Read the model definition and answer for the solid it produces. Units are mm, in the model's axes. Face numbers are marked on the shaded views. A direction names the side the tool comes from. Give positions to 0.01 mm unless a question says otherwise; leave off trailing zeros. Order: outer loops, then holes, each group sorted by start corner. A loop starts at its lowest first (then second) coordinate and runs counter-clockwise, first axis right, second up. Notation, with made-up numbers: (58, 18) - (99, 18) arc R9 cw to (99, 29) - close; hole circle Ø10 at (12.25, 76). An arc over 180 degrees is marked (long way). One line per item, written item: value. Start each with the question number.
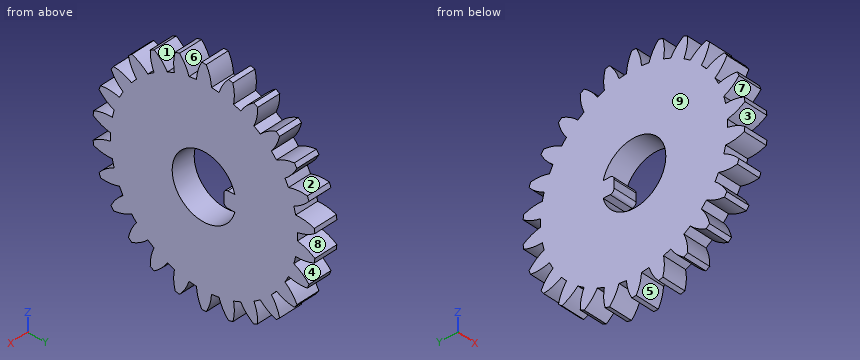
```python
from build123d import *

# Parameters (mm, degrees)
BASPROSKE_W                 = 3
BASPROSKE_H                 = 14
TOOTHCUT_DEPTH              = 21.024984395
TEETHCUTS_COUNT             = 26
TEETHCUTS_ANGLE             = 346.153846154
BORSKE_R                    = 4
BORE_DEPTH                  = 50.0000508
DODANIE_WYCI_GNI_CIE1_DEPTH = 3


with BuildPart() as part:
    # BasProSke → Base-Revolve (revolve)
    with BuildSketch(Plane(origin=(0, 0, 0), x_dir=(1, 0, 0), z_dir=(0, 1, 0)), mode=Mode.PRIVATE) as base_revolve_sk:
        with Locations((1.5, 7)):
            Rectangle(BASPROSKE_W, BASPROSKE_H)
    revolve(base_revolve_sk.sketch.rotate(Axis((-10, 0, 0), (1, 0, 0)), 180), axis=Axis((-10, 0, 0), (1, 0, 0)))

    # TooCutSke → ToothCut (cut, through all)
    with BuildSketch(Plane(origin=(0, 0, 0), x_dir=(0, 0, -1), z_dir=(1, 0, 0))):
        with BuildLine():
            ThreePointArc((0.476965065, 11.739314517), (0, 11.749), (-0.476965065, 11.739314517))
            ThreePointArc((-0.476965065, 11.739314517), (-0.82065865, 12.901686978), (-1.424117301, 13.952911348))
            ThreePointArc((-1.424117301, 13.952911348), (0, 14.0254), (1.424117301, 13.952911348))
            ThreePointArc((1.424117301, 13.952911348), (0.82065865, 12.901686978), (0.476965065, 11.739314517))
        make_face()
    toothcut = extrude(amount=TOOTHCUT_DEPTH, mode=Mode.SUBTRACT)

    # TeethCuts: ToothCut ×26 about axis
    teethcuts_axis = Axis((-10, 0, 0), (1, 0, 0))
    for i in range(1, TEETHCUTS_COUNT):
        add(toothcut.rotate(teethcuts_axis, i * TEETHCUTS_ANGLE / (TEETHCUTS_COUNT - 1)), mode=Mode.SUBTRACT)

    # BorSke → Bore (cut, symmetric)
    with BuildSketch(Plane(origin=(0, 0, 0), x_dir=(0, 0, -1), z_dir=(1, 0, 0))):
        with Locations(Location((0, 0, 0), (0, 0, 180))):
            Circle(BORSKE_R)
    extrude(amount=BORE_DEPTH, both=True, mode=Mode.SUBTRACT)

    # Szkic1 → Dodanie-wyciągnięcie1 (add)
    with BuildSketch(Plane(origin=(3, 0, 0), x_dir=(0, 0, -1), z_dir=(1, 0, 0))):
        with BuildLine():
            Line((0, 4), (-1, 4))
            Line((-1, 4), (-1, 3))
            ThreePointArc((-1, 3), (-0.853553391, 2.646446609), (-0.5, 2.5))
            Line((-0.5, 2.5), (0.5, 2.5))
            ThreePointArc((0.5, 2.5), (0.853553391, 2.646446609), (1, 3))
            Line((1, 3), (1, 4))
            Line((1, 4), (0, 4))
        make_face()
    extrude(amount=-DODANIE_WYCI_GNI_CIE1_DEPTH)


solid = part.part
```
1) Section A-A on z = 0 is taken. Write down the section's boundary in (x, y), plus the area to 3 significant figures.
2) Each of these flat-tipped pins is pushed along its axis until it touches: pin 1 (5 mm diameter, centred on y = 7, z = -5, fed in from -X); pin 2 (0.7 mm diameter, centred on x = 2, y = 3.5, fed in from -Z); pin 3 (0.8 mm diameter, centred on x = 1.5, z = 0, fed in from -Y); pin 4 (1 mm diameter, centred on x = 2, y = 3.5, fed in from +Z). Where does it stop, or does it pass through?
3) Section B-B on z = 6.5 is taken. Write down the section's boundary in (x, y), plus the area to 3 significant figures.
4) Section C-C on z = -7 is taken. Write down the section's boundary in (x, y), plus the area to 3 significant figures.
5) For the marked faces 1, 2, 3, 4 and 5, determine the directions among +Z, -Z, +X, -X, +Y, -Y from which every point of the face is accessible in a straight line to the end or side of a thin tool.
6) The mould has two halves that part along Y. Classify the marked faces 6, 7, 8 and 9: +Y half, -Y half, draft (parallel to the pull), parting line (faces both ways), or undercut.
7) Find the intervals of material crossed by probe 1 along Z at (x, y) = (1.2, 0); probe 2 along Y at (x, z) = (2.1, 0); probe 3 along Z at (x, y) = (1.25, 12.75), in increasing order. Write a range as from..to.
Solved:
1. outline: (0, -11.75) - (3, -11.75) - (3, -4) - (0, -4) - close; (0, 2.5) - (3, 2.5) - (3, 11.75) - (0, 11.75) - close
1. area: 51.0 mm2
2. pin 1: stops at x = 0
2. pin 2: stops at z = -13.64
2. pin 3: stops at y = -11.75
2. pin 4: stops at z = 13.66
3. outline: (0, -10.85) - (3, -10.85) - (3, 10.85) - (0, 10.85) - close
3. area: 65.1 mm2
4. outline: (0, -11.25) - (3, -11.25) - (3, 11.25) - (0, 11.25) - close
4. area: 67.5 mm2
5. face 1: +Z, +X, -X
5. face 2: +X, -X
5. face 3: +X, -X, -Y
5. face 4: +X, -X, +Y
5. face 5: -Z, +X, -X
6. face 6: undercut
6. face 7: -Y half
6. face 8: +Y half
6. face 9: draft
7. probe 1: z = -14..-4, 4..14
7. probe 2: y = -11.75..-4, 2.5..11.75
7. probe 3: z = -5.26..-4.24, -2.29..-0.76, 0.76..2.29, 4.24..5.26
